Source: CAD feature listing. Evaluate the final solid. Frame: model axes, mm. A direction names the side the tool comes from. Round coordinates to 2 decimals unless told otherwise and drop trailing zeros. Loops run counter-clockwise (first coordinate to the right, second up) from the corner with the lowest first, then second, coordinate; pieces in that order, holes last. Notation, with made-up numbers: M 61.5,65.5 L 100.5,65.5 A16 ccw 100.5,70.5 Z; hole C -35.5,24 d2. An arc over 180 degrees is marked long. Write each question's results on one line, items separated by ' | '. Start each with the question number.
1. Section D-D on x = 26.5. Output: boundary loops of the cut face in (y, z).
2. Section C-C on z = 14.75. Output: boundary loops of the cut face in (x, y), and give its area (3 significant figures).
3. Ray query, line 1 (Y direction, x = 107.5, z = 8.5); line 2 (Y direction, x = 141.5, z = 1.75); line 3 (Z direction, x = 125, y = -16.5). Return the intervals inside material, ascending.
4. Contact query for flat-ended pins moving along their axis: pin 1 Ø0.8 at (x, z) = (180, 1.5) entering from -Y; pin 2 Ø10 at (y, z) = (-27, 3.5) entering from -X; pin 3 Ø0.9 at (y, z) = (-38, 4.5) entering from +X; pin 4 Ø5 at (x, y) = (52.51, -14.27) entering from -Z. Output: stop coordinate, or through.
5. Draft query along X for faces 5 (the flat face through (112, -56.852, 9)), 6 (the flat face through (113, -53.852, 9)), 7 (the cylindrical face through (150.097, -36.478, 8.628)), 8 (the flat face through (48.15, -33.82, 10.15)). Return one class per face: released by +X, released by -X, zero draft, split by the parting line, or undercut.
6. Section B-B on x = 88. Output: boundary loops of the cut face in (y, z).
7. Set-up query: faces 1 (the flat face through (65, -6, 17.5)), 2 (the flat face through (154.101, 8, 5)), 3 (the flat face through (113, -19.852, 7)), 4 (the flat face through (66, -43.5, 11)). Return all of +Z, -Z, +X, -X, +Y, -Y with unobstructed straight access to the full face (end or side cutting, diameter ignored); none if empty.
8. Section A-A on y = 24.65. Output: boundary loops of the cut face in (x, z).
from build123d import *

# Parameters (mm, degrees)
EXTRUDE_1_DEPTH     = 2.5
EXTRUDE_2_DEPTH     = 17.5
CUT_EXTRUDE_2_REACH = 212.718
SKETCH_5_W          = 20
SKETCH_5_H          = 5
CHAMFER_1_SIZE      = 1.5
EXTRUDE_3_DEPTH     = 7.5
CUT_EXTRUDE_3_DEPTH = 3
SKETCH_13_R         = 2.5
CUT_EXTRUDE_4_DEPTH = 10
SKETCH_14_W         = 8
SKETCH_14_H         = 15
CUT_EXTRUDE_5_DEPTH = 3
CHAMFER_2_SIZE      = 1
CUT_EXTRUDE_6_REACH = 210.439
SKETCH_15_R         = 4
FILLET_1_R          = 1
CUT_EXTRUDE_7_REACH = 210.669
SKETCH_18_R         = 2.5


with BuildPart() as part:
    # 스케치2 → 보스-돌출1 (new body)
    with BuildSketch(Plane.XY):
        with BuildLine():
            Line((70.1, 38), (0, 38))
            Line((0, 38), (0, 8))
            Line((0, 8), (38.730142729, 8))
            Line((38.730142729, 8), (38.730142729, -24.4))
            Line((38.730142729, -24.4), (57.830142729, -43.5))
            Line((57.830142729, -43.5), (74.630142729, -43.5))
            ThreePointArc((74.630142729, -43.5), (81.464191763, -52.855667895), (92.338911336, -56.852319262))
            Line((92.338911336, -56.852319262), (131.588043415, -56.852319262))
            ThreePointArc((131.588043415, -56.852319262), (144.135794003, -53.569804808), (152.310142729, -43.5))
            Line((152.310142729, -43.5), (168.460142729, -40.652319262))
            Line((168.460142729, -40.652319262), (168.460142729, -15.852319262))
            Line((168.460142729, -15.852319262), (200, -15.852319262))
            Line((200, -15.852319262), (200, 44.147680738))
            Line((200, 44.147680738), (82.3, 44.147680738))
            Line((82.3, 44.147680738), (70.1, 38))
        make_face()
        with BuildLine():
            Line((93.10095722, -19.852319262), (133.10095722, -19.852319262))
            ThreePointArc((133.10095722, -19.852319262), (150.10095722, -36.852319262), (133.10095722, -53.852319262))
            Line((133.10095722, -53.852319262), (93.10095722, -53.852319262))
            ThreePointArc((93.10095722, -53.852319262), (76.10095722, -36.852319262), (93.10095722, -19.852319262))
        make_face(mode=Mode.SUBTRACT)
    extrude(amount=EXTRUDE_1_DEPTH)

    # 스케치2<3> → 보스-돌출2 (add)
    with BuildSketch(Plane.XY):
        with BuildLine():
            Line((70.1, 38), (0, 38))
            Line((0, 38), (0, 8))
            Line((0, 8), (38.730142729, 8))
            Line((38.730142729, 8), (38.730142729, -24.4))
            Line((38.730142729, -24.4), (57.830142729, -43.5))
            Line((57.830142729, -43.5), (74.630142729, -43.5))
            ThreePointArc((74.630142729, -43.5), (81.464191763, -52.855667895), (92.338911336, -56.852319262))
            Line((92.338911336, -56.852319262), (131.588043415, -56.852319262))
            ThreePointArc((131.588043415, -56.852319262), (144.135794003, -53.569804808), (152.310142729, -43.5))
            Line((152.310142729, -43.5), (168.460142729, -40.652319262))
            Line((168.460142729, -40.652319262), (168.460142729, -15.852319262))
            Line((168.460142729, -15.852319262), (70.10095722, -15.852319262))
            Line((70.10095722, -15.852319262), (70.1, 38))
        make_face()
        with BuildLine():
            Line((93.10095722, -19.852319262), (133.10095722, -19.852319262))
            ThreePointArc((133.10095722, -19.852319262), (150.10095722, -36.852319262), (133.10095722, -53.852319262))
            Line((133.10095722, -53.852319262), (93.10095722, -53.852319262))
            ThreePointArc((93.10095722, -53.852319262), (76.10095722, -36.852319262), (93.10095722, -19.852319262))
        make_face(mode=Mode.SUBTRACT)
    extrude(amount=EXTRUDE_2_DEPTH)

    # 스케치5 → 컷-돌출2 (cut, up to next)
    with BuildSketch(Plane.XZ.offset(19.852319262), mode=Mode.PRIVATE) as cut_extrude_2_sk1:
        with Locations((115.10095722, 15)):
            Rectangle(SKETCH_5_W, SKETCH_5_H)
    cut_extrude_2_tool1 = extrude(cut_extrude_2_sk1.sketch, amount=-CUT_EXTRUDE_2_REACH, mode=Mode.PRIVATE) & part.part
    add(cut_extrude_2_tool1.solids().sort_by_distance((115.100957, -19.852319, 15))[0], mode=Mode.SUBTRACT)

    # 모따기1
    chamfer_1_edges = [part.edges().sort_by_distance(p)[0] for p in [
        (125.10095722, -19.852319262, 15),
        (105.10095722, -19.852319262, 15),
    ]]
    chamfer(chamfer_1_edges, length=CHAMFER_1_SIZE)

    # 스케치2<4> → 보스-돌출3 (add)
    with BuildSketch(Plane.XY):
        Polygon((154.10095722, 33.295670157), (70.100083619, 33.295670157), (70.100462148, 12), (70.10095722, -15.852319262), (154.10095722, -15.852319262), align=None)
    extrude(amount=EXTRUDE_3_DEPTH)

    # 스케치2<5> → 컷-돌출3 (cut)
    with BuildSketch(Plane.XY):
        Polygon((66.230142729, 0), (38.730142729, 0), (38.730142729, -24.4), (57.830142729, -43.5), (66.230142729, -43.5), align=None)
    extrude(amount=CUT_EXTRUDE_3_DEPTH, mode=Mode.SUBTRACT)

    # 스케치13 → 컷-돌출4 (cut, symmetric)
    with BuildSketch(Plane.XY.offset(7.5)):
        with Locations((80.6, 9.15)):
            Circle(SKETCH_13_R)
        with Locations((135.59886794, -2.35)):
            Circle(SKETCH_13_R)
        with Locations((142.79886794, 24.65)):
            Circle(SKETCH_13_R)
    extrude(amount=CUT_EXTRUDE_4_DEPTH, both=True, mode=Mode.SUBTRACT)

    # 스케치14 → 컷-돌출5 (cut)
    with BuildSketch(Plane(origin=(0, 0, 3), x_dir=(-1, 0, 0), z_dir=(0, 0, -1))):
        with Locations((-62.230142729, -36)):
            Rectangle(SKETCH_14_W, SKETCH_14_H)
    extrude(amount=-CUT_EXTRUDE_5_DEPTH, mode=Mode.SUBTRACT)

    # 모따기2
    # the kernel refuses this chamfer: 1 mm, written as the material it takes off along each edge
    with BuildSketch(Plane(origin=(58.230142729, -43.5, 0.428317012), x_dir=(-0.9996219169112968, -0.027495876610589005, 0), z_dir=(0, 0, 1))) as chamfer_2_piece_1:
        Polygon((CHAMFER_2_SIZE * 0.999621916911, -CHAMFER_2_SIZE * 0.0274958766106), (-CHAMFER_2_SIZE * 0.0274958766106, -CHAMFER_2_SIZE * 0.999621916911), (0, 0), align=None)
    extrude(amount=5.571682988, mode=Mode.SUBTRACT)

    # 스케치15 → 컷-돌출6 (cut, up to next)
    with BuildSketch(Plane(origin=(0, 0, 3), x_dir=(-1, 0, 0), z_dir=(0, 0, -1)), mode=Mode.PRIVATE) as cut_extrude_6_sk1:
        with Locations((-52.505609521, -14.268427339)):
            Circle(SKETCH_15_R)
    cut_extrude_6_tool1 = extrude(cut_extrude_6_sk1.sketch, amount=-CUT_EXTRUDE_6_REACH, mode=Mode.PRIVATE) & part.part
    add(cut_extrude_6_tool1.solids().sort_by_distance((52.50561, -14.268427, 3))[0], mode=Mode.SUBTRACT)

    # 필렛1
    fillet_1_edges = [part.edges().sort_by_distance(p)[0] for p in [
        (56.505609521, -14.268427339, 3),
    ]]
    fillet(fillet_1_edges, radius=FILLET_1_R)

    # 스케치18 → 컷-돌출7 (cut, up to next)
    with BuildSketch(Plane(origin=(0, 0, 0), x_dir=(-1, 0, 0), z_dir=(0, 0, -1)), mode=Mode.PRIVATE) as cut_extrude_7_sk1:
        with Locations((-160.302780776, -29.676087823)):
            Circle(SKETCH_18_R)
    cut_extrude_7_tool1 = extrude(cut_extrude_7_sk1.sketch, amount=-CUT_EXTRUDE_7_REACH, mode=Mode.PRIVATE) & part.part
    add(cut_extrude_7_tool1.solids().sort_by_distance((160.302781, -29.676088, 0))[0], mode=Mode.SUBTRACT)


solid = part.part
Taken from the geometry:
1) outline: M 8,0 L 38,0 L 38,17.5 L 8,17.5 Z
2) outline: M 0,8 L 38.73,8 L 38.73,-24.4 L 57.83,-43.5 L 74.63,-43.5 A20 ccw 92.34,-56.85 L 131.59,-56.85 A20.83 ccw 152.31,-43.5 L 168.46,-40.65 L 168.46,-15.85 L 125.1,-15.85 L 125.1,-18.35 L 126.6,-19.85 L 133.1,-19.85 A17 cw 133.1,-53.85 L 93.1,-53.85 A17 cw 93.1,-19.85 L 103.6,-19.85 L 105.1,-18.35 L 105.1,-15.85 L 70.1,-15.85 L 70.1,38 L 0,38 Z; hole C 52.51,-14.27 d8; hole C 160.3,-29.68 d5 | area: 4,710 mm^2
3) line 1: -56.85 to -53.85, -19.85 to -15.85 | line 2: -55.01 to -51.63, -22.07 to 22.51, 26.79 to 44.15 | line 3: 0 to 12.5
4) pin 1: y = -15.85 | pin 2: x = 38.73 | pin 3: x = 168.46 | pin 4: through
5) face 5: zero draft | face 6: undercut | face 7: undercut | face 8: released by -X
6) outline: M -56.11,0 L -53.07,0 L -53.07,17.5 L -56.11,17.5 Z; M -20.64,0 L 44.15,0 L 44.15,2.5 L 33.3,2.5 L 33.3,7.5 L -15.85,7.5 L -15.85,17.5 L -20.64,17.5 Z
7) face 1: +Z, +X, -X, +Y, -Y | face 2: +Z, +X, +Y | face 3: +Z, -Z | face 4: +Z, -Z, -X, -Y
8) outline: M 0,0 L 140.3,0 L 140.3,7.5 L 70.1,7.5 L 70.1,17.5 L 0,17.5 Z; M 145.3,0 L 200,0 L 200,2.5 L 154.1,2.5 L 154.1,7.5 L 145.3,7.5 Z
